Geometry check sheet. Reference: the model listing, model coordinates, mm. Face numbers are marked on the shaded views. A direction names the side the tool comes from. Coordinates: 2 decimals unless noted, no trailing zeros. Loops run counter-clockwise (first coordinate to the right, second up) from the corner with the lowest first, then second, coordinate; pieces in that order, holes last. Notation, with made-up numbers: (69, 67) - (106, 67) arc R16 cw to (106, 75) - close; hole circle Ø2 at (85.5, 22). An arc over 180 degrees is marked (long way). One line per item, written item: value.
from build123d import *

# Parameters (mm, degrees)
SKETCH_1_R           = 11.75
SKETCH_1_R_2         = 1.6
EXTRUDE_1_DEPTH      = 3
M3X0_5_4_D           = 2.5
M3X0_5_4_CSINK_D     = 3.05
M3X0_5_4_CSINK_ANGLE = 90
M4X0_7_1_D           = 3.3
M4X0_7_1_CSINK_D     = 4.05
M4X0_7_1_CSINK_ANGLE = 90
M3X0_5_5_D           = 2.5
M3X0_5_5_CSINK_D     = 3.05
M3X0_5_5_CSINK_ANGLE = 90
SKETCH_23_W          = 9.6
SKETCH_23_H          = 20.5
SKETCH_23_W_2        = 2.4
SKETCH_23_W_3        = 4
CUT_EXTRUDE_4_DEPTH  = 1.2
FILLET_1_R           = 0.6


with BuildPart() as part:
    # 草图1 → 凸台-拉伸1 (new body)
    with BuildSketch(Plane.XY):
        with BuildLine():
            Line((-30, -25), (-30, -67))
            ThreePointArc((-30, -67), (-29.121320344, -69.121320344), (-27, -70))
            Line((-27, -70), (27, -70))
            ThreePointArc((27, -70), (29.121320344, -69.121320344), (30, -67))
            Line((30, -67), (30, 22))
            ThreePointArc((30, 22), (29.121320344, 24.121320344), (27, 25))
            Line((27, 25), (-27, 25))
            ThreePointArc((-27, 25), (-29.121320344, 24.121320344), (-30, 22))
            Line((-30, 22), (-30, -25))
        make_face()
        with Locations((0, 5)):
            Circle(SKETCH_1_R, mode=Mode.SUBTRACT)
        with Locations((15.5, 20.5)):
            Circle(SKETCH_1_R_2, mode=Mode.SUBTRACT)
        with Locations((-15.5, 20.5)):
            Circle(SKETCH_1_R_2, mode=Mode.SUBTRACT)
        with Locations((-15.5, -10.5)):
            Circle(SKETCH_1_R_2, mode=Mode.SUBTRACT)
        with Locations((15.5, -10.5)):
            Circle(SKETCH_1_R_2, mode=Mode.SUBTRACT)
        with Locations((-8, -30)):
            Circle(SKETCH_1_R_2, mode=Mode.SUBTRACT)
        with Locations((8, -30)):
            Circle(SKETCH_1_R_2, mode=Mode.SUBTRACT)
        with Locations((-8, -45)):
            Circle(SKETCH_1_R_2, mode=Mode.SUBTRACT)
        with Locations((8, -45)):
            Circle(SKETCH_1_R_2, mode=Mode.SUBTRACT)
    extrude(amount=EXTRUDE_1_DEPTH)

    # M3x0.5 螺纹孔4 (through all)
    with Locations(Plane.XY.offset(3)):
        with Locations((-25, -44), (-25, -54), (25, -44), (25, -54), (25, -64), (-25, -64), (-8, -14), (8, -14), (25, -34), (-25, -34), (-25, -24)):
            CounterSinkHole(M3X0_5_4_D / 2, M3X0_5_4_CSINK_D / 2, counter_sink_angle=M3X0_5_4_CSINK_ANGLE)

    # M4x0.7 螺纹孔1 (through all)
    with Locations(Plane(origin=(0, 0, 0), x_dir=(-1, 0, 0), z_dir=(0, 0, -1))):
        with Locations((0, -55), (0, -64.5)):
            CounterSinkHole(M4X0_7_1_D / 2, M4X0_7_1_CSINK_D / 2, counter_sink_angle=M4X0_7_1_CSINK_ANGLE)

    # M3x0.5 螺纹孔5 (through all)
    with Locations(Plane(origin=(0, 0, 0), x_dir=(-1, 0, 0), z_dir=(0, 0, -1))):
        with Locations((-25, 20), (25, 20)):
            CounterSinkHole(M3X0_5_5_D / 2, M3X0_5_5_CSINK_D / 2, counter_sink_angle=M3X0_5_5_CSINK_ANGLE)

    # 草图23 → 切除-拉伸4 (cut)
    with BuildSketch(Plane(origin=(0, 0, 0), x_dir=(-1, 0, 0), z_dir=(0, 0, -1))):
        with Locations((-25.2, -59.75)):
            Rectangle(SKETCH_23_W, SKETCH_23_H)
        with Locations((25.2, -59.75)):
            Rectangle(SKETCH_23_W, SKETCH_23_H)
        with Locations((-18.4, -59.75)):
            Rectangle(SKETCH_23_W_2, SKETCH_23_H)
        with Locations((-15.2, -59.75)):
            Rectangle(SKETCH_23_W_2, SKETCH_23_H)
        with Locations((-12, -59.75)):
            Rectangle(SKETCH_23_W_2, SKETCH_23_H)
        with Locations((-8, -59.75)):
            Rectangle(SKETCH_23_W_3, SKETCH_23_H)
        with Locations((12, -59.75)):
            Rectangle(SKETCH_23_W_2, SKETCH_23_H)
        with Locations((8, -59.75)):
            Rectangle(SKETCH_23_W_3, SKETCH_23_H)
        with Locations((15.2, -59.75)):
            Rectangle(SKETCH_23_W_2, SKETCH_23_H)
        with Locations((18.4, -59.75)):
            Rectangle(SKETCH_23_W_2, SKETCH_23_H)
    extrude(amount=-CUT_EXTRUDE_4_DEPTH, mode=Mode.SUBTRACT)

    # 圆角1
    fillet_1_edges = [part.edges().sort_by_distance(p)[0] for p in [
        (20.4, -49.5, 0.6),
        (-17.2, -49.5, 0.6),
        (-19.6, -49.5, 0.6),
        (13.2, -49.5, 0.6),
        (10.8, -49.5, 0.6),
        (16.4, -49.5, 0.6),
        (14, -49.5, 0.6),
        (19.6, -49.5, 0.6),
        (17.2, -49.5, 0.6),
        (-20.4, -49.5, 0.6),
        (-14, -49.5, 0.6),
        (-16.4, -49.5, 0.6),
        (-6, -49.5, 0.6),
        (-10, -49.5, 0.6),
        (-10.8, -49.5, 0.6),
        (-13.2, -49.5, 0.6),
        (10, -49.5, 0.6),
        (6, -49.5, 0.6),
    ]]
    fillet(fillet_1_edges, radius=FILLET_1_R)


solid = part.part
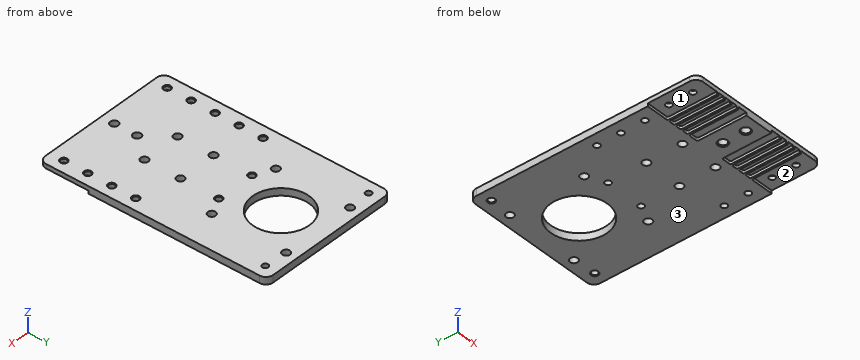
(1) Material ranges on probe 1 along Y at (x, z) = (25, 1.6); probe 2 along Y at (x, z) = (0, 1.5); probe 3 along X at (y, z) = (-55, 1.45), recorded low to high. Write a range as from..to.
Reply:
probe 1: -70..-65.25, -62.75..-55.25, -52.75..-45.25, -42.75..-35.25, -32.75..18.75, 21.25..25
probe 2: -70..-66.15, -62.85..-56.65, -53.35..-6.75, 16.75..25
probe 3: -30..-25.75, -24.25..-1.65, 1.65..24.25, 25.75..30
(2) Cross-section at B-B on z = 2.1. State how many separate pieces and enclosed holes the cut face has, and give its area (3 significant figures).
Reply:
separate pieces: 1
enclosed holes: 24
area: 5,110 mm2
(3) Access from +Z, -Z, +X, -X, +Y, -Y to the whole of each face (thin tool, end or side, straight path). Record for the marked faces 1, 2 and 3.
Reply:
face 1: -Z, -X, -Y
face 2: -Z, +X, -Y
face 3: -Z, +X, -X, +Y, -Y
(4) Cross-section at A-A on y = -34. Record the cut outline in (x, z) (3 decimals), and give its area (3 significant figures).
Reply:
outline: (-30, 0) - (-26.25, 0) - (-26.25, 2.725) - (-26.525, 3) - (-30, 3) - close; (-23.75, 0) - (23.75, 0) - (23.75, 2.725) - (23.475, 3) - (-23.475, 3) - (-23.75, 2.725) - close; (26.25, 0) - (30, 0) - (30, 3) - (26.525, 3) - (26.25, 2.725) - close
area: 165 mm2
(5) Go/stop test with flat-tipped pins: pin 1 Ø1.2 at (x, y) = (12.5, -56.5) entering from -Z; pin 2 Ø3 at (x, y) = (25, -44) entering from +Z (3 decimals). Record where each tip stops, or that it passes through.
Reply:
pin 1: z = 1.2
pin 2: z = 2.975
